Geometry check sheet. Reference: the model listing, model coordinates, mm. A direction names the side the tool comes from. Round coordinates to 2 decimals unless told otherwise and drop trailing zeros. Write each loop counter-clockwise with the first axis right and the second up, starting at its lowest first coordinate (ties: lowest second). Pieces come first, ordered by that corner, then holes. Notation, with made-up numbers: (78.25, 80) - (118.25, 80) arc R25 ccw to (118.25, 118) - close; hole circle Ø4 at (40.25, -19). An arc over 180 degrees is marked (long way). Return JSON: item names as keys, results as strings. Group by question number.
Autodesk Inventor part; units mm, degrees
ref_plane "YZ Plane" through (0, 0, 0) normal (1, 0, 0) x (0, 1, 0)
ref_plane "XZ Plane" through (0, 0, 0) normal (0, 1, 0) x (-1, 0, 0)
ref_plane "XY Plane" through (0, 0, 0) normal (0, 0, 1) x (1, 0, 0)
sketch "Sketch2" plane through (0, 0, 0) normal (0, 0, 1) x (1, 0, 0)
  line L0 (0, 0) -> (-101.6, 0)
  line L1 (-101.6, 0) -> (-101.6, 101.6)
  line L2 (-101.6, 101.6) -> (0, 101.6)
  line L3 (0, 101.6) -> (0, 0)
  circle A0 centre (-12.7, 88.9) radius 2.5797
  circle A1 centre (-50.8, 76.2) radius 9.525
  circle A2 centre (-25.4, 38.1) radius 2.5797
  circle A3 centre (-50.8, 25.4) radius 9.525
  circle A4 centre (-88.9, 88.9) radius 2.5797
  circle A5 centre (-12.7, 63.5) radius 2.5797
  circle A6 centre (-88.9, 63.5) radius 2.5797
  circle A7 centre (-76.2, 38.1) radius 2.5797
  circle A8 centre (-25.4, 12.7) radius 2.5797
  circle A9 centre (-76.2, 12.7) radius 2.5797
  line L4 (-85.725, 19.05) -> (-101.6, 19.05)
  line L5 (-101.6, 19.05) -> (-101.6, 22.225)
  line L6 (-101.6, 22.225) -> (-85.725, 22.225)
  line L7 (-85.725, 22.225) -> (-85.725, 19.05)
  line L8 (-101.6, 22.225) -> (-85.725, 22.225)
  line L9 (-85.725, 22.225) -> (-85.725, 23.8125)
  line L10 (-85.725, 23.8125) -> (-101.6, 23.8125)
  line L11 (-101.6, 23.8125) -> (-101.6, 22.225)
  line L12 (-85.725, 23.8125) -> (-101.6, 23.8125)
  line L13 (-101.6, 23.8125) -> (-101.6, 26.9875)
  line L14 (-101.6, 26.9875) -> (-85.725, 26.9875)
  line L15 (-85.725, 26.9875) -> (-85.725, 23.8125)
  line L16 (-101.6, 26.9875) -> (-85.725, 26.9875)
  line L17 (-85.725, 26.9875) -> (-85.725, 28.575)
  line L18 (-85.725, 28.575) -> (-101.6, 28.575)
  line L19 (-101.6, 28.575) -> (-101.6, 26.9875)
  line L20 (-85.725, 28.575) -> (-101.6, 28.575)
  line L21 (-101.6, 28.575) -> (-101.6, 31.75)
  line L22 (-101.6, 31.75) -> (-85.725, 31.75)
  line L23 (-85.725, 31.75) -> (-85.725, 28.575)
  line L24 (-85.725, 31.8135) -> (-101.6, 31.8135)
  line L25 (-101.6, 31.8135) -> (-101.6, 28.5115)
  line L26 (-101.6, 28.5115) -> (-85.725, 28.5115)
  line L27 (-85.725, 28.5115) -> (-85.725, 31.8135)
  line L28 (-85.725, 27.051) -> (-101.6, 27.051)
  line L29 (-101.6, 27.051) -> (-101.6, 23.749)
  line L30 (-101.6, 23.749) -> (-85.725, 23.749)
  line L31 (-85.725, 23.749) -> (-85.725, 27.051)
  line L32 (-85.725, 22.2885) -> (-101.6, 22.2885)
  line L33 (-101.6, 22.2885) -> (-101.6, 18.9865)
  line L34 (-101.6, 18.9865) -> (-85.725, 18.9865)
  line L35 (-85.725, 18.9865) -> (-85.725, 22.2885)
  line L36 (-101.6, 26.4583) -> (-85.725, 26.4583)
  line L37 (-85.725, 26.4583) -> (-85.725, 24.3417)
  line L38 (-85.725, 24.3417) -> (-101.6, 24.3417)
  line L39 (-101.6, 24.3417) -> (-101.6, 26.4583)
  line L40 (-50.8, 0) -> (-50.8, 101.6)
  line L41 (-15.875, 19.05) -> (0, 19.05)
  line L42 (0, 19.05) -> (0, 22.225)
  line L43 (0, 22.225) -> (-15.875, 22.225)
  line L44 (-15.875, 22.225) -> (-15.875, 19.05)
  line L45 (0, 22.225) -> (-15.875, 22.225)
  line L46 (-15.875, 22.225) -> (-15.875, 23.8125)
  line L47 (-15.875, 23.8125) -> (0, 23.8125)
  line L48 (0, 23.8125) -> (0, 22.225)
  line L49 (-15.875, 23.8125) -> (0, 23.8125)
  line L50 (0, 23.8125) -> (0, 26.9875)
  line L51 (0, 26.9875) -> (-15.875, 26.9875)
  line L52 (-15.875, 26.9875) -> (-15.875, 23.8125)
  line L53 (0, 26.9875) -> (-15.875, 26.9875)
  line L54 (-15.875, 26.9875) -> (-15.875, 28.575)
  line L55 (-15.875, 28.575) -> (0, 28.575)
  line L56 (0, 28.575) -> (0, 26.9875)
  line L57 (-15.875, 28.575) -> (0, 28.575)
  line L58 (0, 28.575) -> (0, 31.75)
  line L59 (0, 31.75) -> (-15.875, 31.75)
  line L60 (-15.875, 31.75) -> (-15.875, 28.575)
  line L61 (-15.875, 31.8135) -> (0, 31.8135)
  line L62 (0, 31.8135) -> (0, 28.5115)
  line L63 (0, 28.5115) -> (-15.875, 28.5115)
  line L64 (-15.875, 28.5115) -> (-15.875, 31.8135)
  line L65 (-15.875, 27.051) -> (0, 27.051)
  line L66 (0, 27.051) -> (0, 23.749)
  line L67 (0, 23.749) -> (-15.875, 23.749)
  line L68 (-15.875, 23.749) -> (-15.875, 27.051)
  line L69 (-15.875, 22.2885) -> (0, 22.2885)
  line L70 (0, 22.2885) -> (0, 18.9865)
  line L71 (0, 18.9865) -> (-15.875, 18.9865)
  line L72 (-15.875, 18.9865) -> (-15.875, 22.2885)
  line L73 (0, 26.4583) -> (-15.875, 26.4583)
  line L74 (-15.875, 26.4583) -> (-15.875, 24.3417)
  line L75 (-15.875, 24.3417) -> (0, 24.3417)
  line L76 (0, 24.3417) -> (0, 26.4583)
  point P0 (-101.6, 30.1625)
  point P1 (-101.6, 20.6375)
  point P2 (-101.6, 25.4)
  point P3 (-85.725, 25.4)
  point P4 (0, 30.1625)
  point P5 (0, 20.6375)
  point P6 (0, 25.4)
  point P7 (-15.875, 25.4)
  point P8 (-50.8, 15.875)
  point P9 (-50.8, 34.925)
  point P10 (-50.8, 66.675)
  point P11 (-50.8, 85.725)
  dimension "d60" = 101.6
  dimension "d61" = 101.6
  dimension "d62" = 19.05
  dimension "d63" = 5.1594
  dimension "d66" = 12.7
  dimension "d69" = 76.2
  dimension "d72" = 25.4
  dimension "d75" = 12.7
  dimension "d76" = 38.1
  dimension "d77" = 12.7
  dimension "d80" = 50.8
  dimension "d83" = 25.4
  dimension "d86" = 25.4
  dimension "d87" = 12.7
  dimension "d88" = 12.7
  dimension "d89" = 25.4
  dimension "d96" = 3.175
  dimension "d97" = 1.5875
  dimension "d98" = 3.302
  dimension "d101" = 2.1167
  dimension "d103" = 15.875
  dimension "d104" = 25.4
extrude "Extrusion2" add sketch "Sketch2" along normal blind 3.175 contours L0 L40 A3 A1 L2 L3 L61 L64 L60 L54 L52 L46 L44 L72 L71 | L0 L1 L34 L35 L7 L9 L15 L17 L23 L27 L24 L2 L40 A1 A3 | L40 A1 | A1 L40 | L67 L46 L47 L3 | L47 L52 L75 L3 | L1 L10 L9 L30 | L75 L52 L73 L3 | L1 L38 L15 L10 | L73 L52 L51 L3 | L1 L36 L15 L38 | L51 L54 L65 L3 | L1 L14 L15 L36 | L1 L28 L17 L14
fillet "Fillet3" radius 3.175 8 edges at (0, 101.6, 1.5875) (-101.6, 101.6, 1.5875) (0, 18.9865, 1.5875) (0, 31.8135, 1.5875) (0, 0, 1.5875) (-101.6, 0, 1.5875) (-101.6, 18.9865, 1.5875) (-101.6, 31.8135, 1.5875)
fillet "Fillet5" radius 0.7937 4 edges at (0, 27.051, 1.5875) (0, 23.749, 1.5875) (-101.6, 27.051, 1.5875) (-101.6, 23.749, 1.5875)
properties part number "Dipper Plate (backplate)"
1. Section check C-C (x = -50.5). Enter the section's corners in (y, z) (3 decimals).
2. Section check A-A (y = 88.9). Enter the section's corners in (x, z) (3 decimals), and give its area (3 significant figures).
3. Tool access check on faces 1 (the face through (-15.875, 21, 2)), 2 (the face through (-93, 23.749, 2)), 3 (the face through (-51, 101.6, 2)). Record the directions out of +Z, -Z, +X, -X, +Y, -Y that give a thin tool (end or side, any length) a straight path to the whole face; none if there is none.
4. Depth check by flat-ended pin: pin 1 Ø1 at (y, z) = (28.5, 1) entering from -X (3 decimals); pin 2 Ø6 at (x, y) = (-32, 91) entering from -Z; pin 3 Ø1 at (y, z) = (20.5, 1.5) entering from +X (3 decimals). Enter the tip coordinate at first touch or a pass-through.
5. Material ranges on line 1 along Y through (x, z) = (-76.5, 2.3); line 2 along Y through (x, z) = (-12.7, 0.95); line 3 along X through (y, z) = (25.4, 0.75) (3 decimals), recorded low to high.
6. Section check B-B (x = -12.7). Enter the section's corners in (y, z) (1 decimal), and give its area (3 significant figures).
7. Mould release check, pull along Y, two halves, no side actions. Record for faces 4 (the face through (-0.95, 0.91, 1.61)), 5 (the face through (-0.955, 32.719, 1.61)), 6 (the face through (0, 10, 2)): pulls with the +Y half, pulls with the -Y half, needs draft (parallel to the pull), parting line crosses it, or undercut.
8. Section check D-D (z = 1.85). State how many separate pieces and enclosed holes the cut face has, and give its area (3 significant figures).
Result sheet:
{
 "1": {"outline": "(0, 0) - (15.88, 0) - (15.88, 3.175) - (0, 3.175) - close; (34.92, 0) - (101.6, 0) - (101.6, 3.175) - (34.92, 3.175) - close"},
 "2": {"outline": "(-101.6, 0) - (-91.48, 0) - (-91.48, 3.175) - (-101.6, 3.175) - close; (-86.32, 0) - (-15.28, 0) - (-15.28, 3.175) - (-86.32, 3.175) - close; (-10.12, 0) - (0, 0) - (0, 3.175) - (-10.12, 3.175) - close", "area": "290 mm²"},
 "3": {"face 1": "+Z, -Z, +X", "face 2": "+Z, -Z, -X", "face 3": "+Z, -Z, +X, -X, +Y"},
 "4": {"pin 1": "stops at x = -85.725", "pin 2": "stops at z = 0", "pin 3": "stops at x = -15.875"},
 "5": {"line 1": "y = 0 to 10.14, 15.26 to 35.54, 40.66 to 101.6", "line 2": "y = 0 to 18.99, 23.75 to 27.05, 31.81 to 60.92, 66.08 to 86.32, 91.48 to 101.6", "line 3": "x = -101.6 to -60.325, -41.275 to 0"},
 "6": {"outline": "(0, 0) - (19, 0) - (19, 3.2) - (0, 3.2) - close; (23.7, 0) - (27.1, 0) - (27.1, 3.2) - (23.7, 3.2) - close; (31.8, 0) - (60.9, 0) - (60.9, 3.2) - (31.8, 3.2) - close; (66.1, 0) - (86.3, 0) - (86.3, 3.2) - (66.1, 3.2) - close; (91.5, 0) - (101.6, 0) - (101.6, 3.2) - (91.5, 3.2) - close", "area": "260 mm²"},
 "7": {"face 4": "pulls with the -Y half", "face 5": "undercut", "face 6": "needs draft"},
 "8": {"separate pieces": "1", "enclosed holes": "9", "area": "9,550 mm²"}
}
